Verification items for this drawing (mm, ordinates from the low corner). Coordinates: 2 decimals unless noted, no trailing zeros. Order: outer loops, then holes, each group sorted by start corner. A loop starts at its lowest first (then second) coordinate and runs counter-clockwise, first axis right, second up. Notation, with made-up numbers: M 45.5,31 L 49.5,31 A8 ccw 49.5,43 Z; hole C 23.25,37.25 d9. An arc over 180 degrees is marked long. Return JSON: item names as keys, results as strings. Group by question number.
1. Section check D-D, the plane y = 113. Record the cut outline in (x, z).
2. Section check C-C, the plane z = 22. Record the cut outline in (x, y).
3. Gauge pin test, flat ends, axial feed: pin 1 (4 mm diameter, centred on y = 65, z = 39, fed in from +X); pin 2 (1.9 mm diameter, centred on y = 10, z = 22.2, fed in from +X); pin 3 (1.8 mm diameter, centred on x = 7, z = 25, fed in from +Y). Record the tip position at first contact, or that the pin passes through.
4. Mould release check, pull along Z, two halves, no side actions. Record for the marked faces 1, 2, 3 and 4: +Z half, -Z half, draft (parallel to the pull), parting line (faces both ways), or undercut.
5. Material ranges on line 1 along Y through (x, z) = (1.25, 22.2); line 2 along Z through (x, y) = (6.75, 78); line 3 along Z through (x, y) = (2.45, 10), recorded low to high.
6. Section check B-B, the plane x = 3.5. Record the cut outline in (y, z).
7. Section check A-A, the plane y = 10. Record the cut outline in (x, z), plus the area to 3 significant figures.
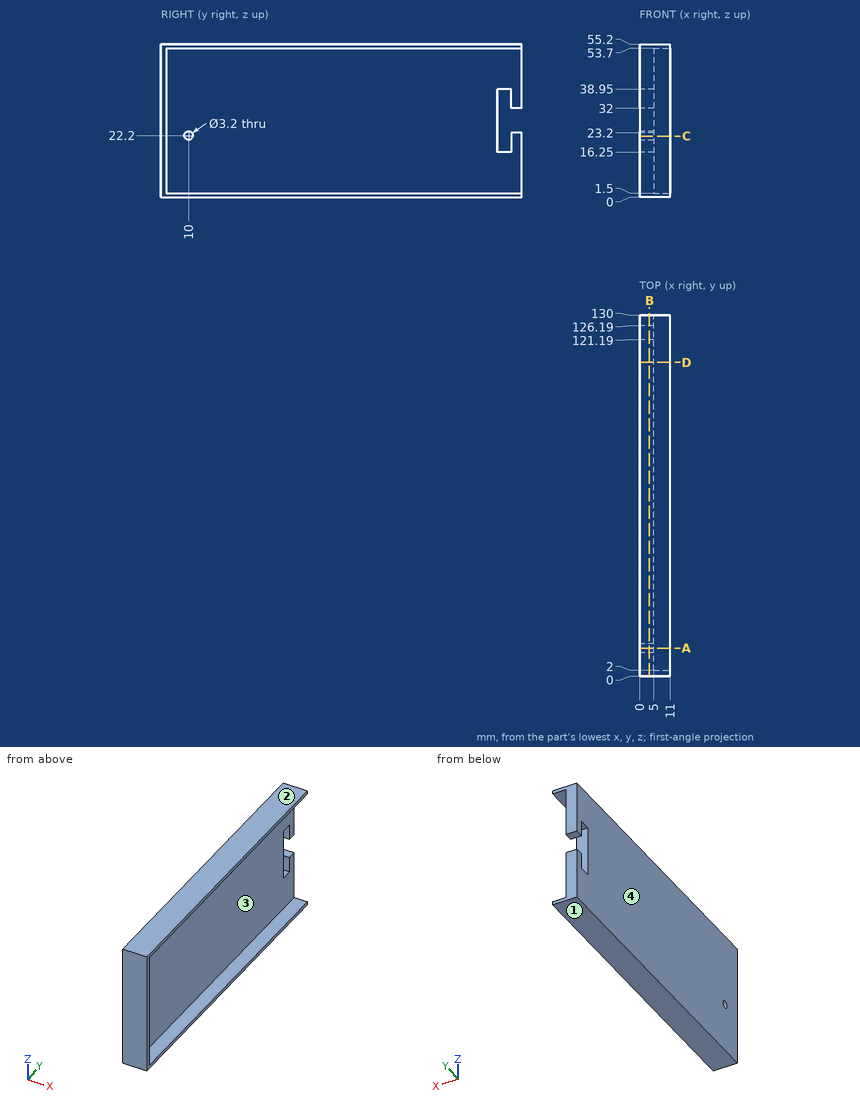
Answers follow:
{
 "1": {"outline": "M 0,0 L 11,0 L 11,1.5 L 5,1.5 L 5,53.7 L 11,53.7 L 11,55.2 L 0,55.2 Z"},
 "2": {"outline": "M 0,0 L 11,0 L 11,2 L 5,2 L 5,8.41 L 0,8.41 Z; M 0,11.59 L 5,11.59 L 5,121.19 L 0,121.19 Z; M 0,126.19 L 5,126.19 L 5,130 L 0,130 Z"},
 "3": {"pin 1": "x = 5", "pin 2": "through", "pin 3": "y = 2"},
 "4": {"face 1": "-Z half", "face 2": "+Z half", "face 3": "undercut", "face 4": "draft"},
 "5": {"line 1": "0 to 8.4, 11.6 to 121.19, 126.19 to 130", "line 2": "0 to 1.5, 53.7 to 55.2", "line 3": "0 to 20.6, 23.8 to 55.2"},
 "6": {"outline": "M 0,0 L 130,0 L 130,23.2 L 126.19,23.2 L 126.19,16.25 L 121.19,16.25 L 121.19,38.95 L 126.19,38.95 L 126.19,32 L 130,32 L 130,55.2 L 0,55.2 Z; hole C 10,22.2 d3.2"},
 "7": {"outline": "M 0,0 L 11,0 L 11,1.5 L 5,1.5 L 5,20.6 L 0,20.6 Z; M 0,23.8 L 5,23.8 L 5,53.7 L 11,53.7 L 11,55.2 L 0,55.2 Z", "area": "278 mm^2"}
}
